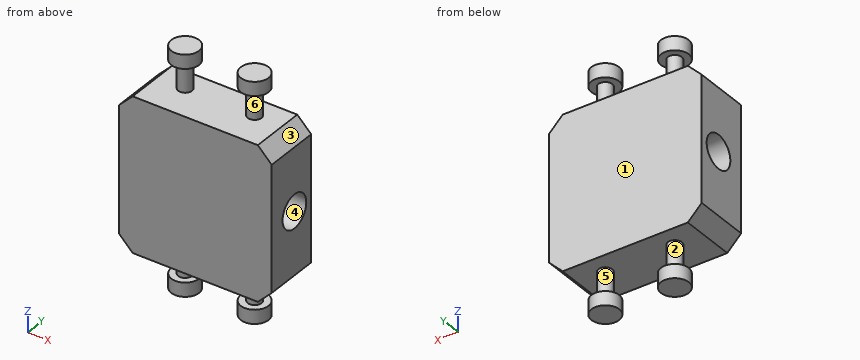
```python
from build123d import *

# Parameters (mm, degrees)
SKETCH2_W           = 110
SKETCH2_H           = 110
BOSS_EXTRUDE1_DEPTH = 30
CHAMFER1_SIZE       = 10
SKETCH3_R           = 5
BOSS_EXTRUDE2_DEPTH = 20
BOSS_EXTRUDE3_START = 20
SKETCH4_R           = 5
BOSS_EXTRUDE3_DEPTH = 20
SKETCH5_R           = 10
BOSS_EXTRUDE4_DEPTH = 10
BOSS_EXTRUDE5_START = 10
SKETCH6_R           = 10
BOSS_EXTRUDE5_DEPTH = 10
BOSS_EXTRUDE6_DEPTH = 5
BOSS_EXTRUDE7_DEPTH = 5
SKETCH15_R          = 12
CUT_EXTRUDE1_DEPTH  = 200


with BuildPart() as part:
    # Sketch2 → Boss-Extrude1 (new body)
    with BuildSketch(Plane(origin=(0, 0, 0), x_dir=(1, 0, 0), z_dir=(0, 1, 0))):
        with Locations((55, 55)):
            Rectangle(SKETCH2_W, SKETCH2_H)
    extrude(amount=BOSS_EXTRUDE1_DEPTH)

    # Chamfer1
    chamfer1_edges = [part.edges().sort_by_distance(p)[0] for p in [
        (0, 15, -110),
        (110, 15, -110),
        (110, 15, 0),
        (0, 15, 0),
    ]]
    chamfer(chamfer1_edges, length=CHAMFER1_SIZE)

    # Sketch3 → Boss-Extrude2 (add)
    with BuildSketch(Plane.XY):
        with Locations(Location((30, 20, 0), (0, 0, 180))):
            Circle(SKETCH3_R)
        with Locations(Location((80, 20, 0), (0, 0, 180))):
            Circle(SKETCH3_R)
    extrude(amount=BOSS_EXTRUDE2_DEPTH)

    # Sketch4 → Boss-Extrude3 (add)
    with BuildSketch(Plane(origin=(0, 0, -110), x_dir=(-1, 0, 0), z_dir=(0, 0, -1)).offset(BOSS_EXTRUDE3_START)):
        with Locations((-80, 20)):
            Circle(SKETCH4_R)
        with Locations((-30, 20)):
            Circle(SKETCH4_R)
    extrude(amount=-BOSS_EXTRUDE3_DEPTH)

    # Sketch5 → Boss-Extrude4 (add)
    with BuildSketch(Plane(origin=(0, 0, -130), x_dir=(-1, 0, 0), z_dir=(0, 0, -1))):
        with Locations((-80, 20)):
            Circle(SKETCH5_R)
        with Locations((-30, 20)):
            Circle(SKETCH5_R)
    extrude(amount=BOSS_EXTRUDE4_DEPTH)

    # Sketch6 → Boss-Extrude5 (add)
    with BuildSketch(Plane.XY.offset(20).offset(BOSS_EXTRUDE5_START)):
        with Locations(Location((30, 20, 0), (0, 0, 180))):
            Circle(SKETCH6_R)
        with Locations(Location((80, 20, 0), (0, 0, 180))):
            Circle(SKETCH6_R)
    extrude(amount=-BOSS_EXTRUDE5_DEPTH)

    # Sketch9 → Boss-Extrude6 (add)
    with BuildSketch(Plane(origin=(0, 30, 0), x_dir=(1, 0, 0), z_dir=(0, 1, 0))):
        Polygon((10, 110), (100, 110), (110, 100), (110, 10), (100, 0), (10, 0), (0, 10), (0, 100), align=None)
    extrude(amount=BOSS_EXTRUDE6_DEPTH)

    # Sketch10 → Boss-Extrude7 (add)
    with BuildSketch(Plane.XZ):
        Polygon((10, 0), (100, 0), (110, -10), (110, -100), (100, -110), (10, -110), (0, -100), (0, -10), align=None)
    extrude(amount=BOSS_EXTRUDE7_DEPTH)

    # Sketch15 → Cut-Extrude1 (cut)
    with BuildSketch(Plane(origin=(110, 0, 0), x_dir=(0, 0, -1), z_dir=(1, 0, 0))):
        with Locations((55, 18)):
            Circle(SKETCH15_R)
    extrude(amount=-CUT_EXTRUDE1_DEPTH, mode=Mode.SUBTRACT)


solid = part.part
```
Geometry: final body of the model. Coordinates: model frame, mm. Face numbers are marked on the shaded views. A direction names the side the tool comes from. Coordinates: 2 decimals unless noted, no trailing zeros. Order: outer loops, then holes, each group sorted by start corner. A loop starts at its lowest first (then second) coordinate and runs counter-clockwise, first axis right, second up. Notation, with made-up numbers: (27.5, -30.75) -> (31.5, -30.75) arc R20 ccw to (31.5, -14.75) -> close; hole circle Ø9 at (71, -22). An arc over 180 degrees is marked (long way). Answer in a Markdown table with one row per item.
Item 1: Section D-D on z = -102.5. Output: boundary loops of the cut face in (x, y).
Return value:
| item | result |
|---|---|
| outline | (2.5, -5) -> (107.5, -5) -> (107.5, 35) -> (2.5, 35) -> close |
Item 2: Draft query along X for the marked faces 3, 4, 5 and 6. Return one class per face: released by +X, released by -X, zero draft, split by the parting line, or undercut.
Return value:
| item | result |
|---|---|
| face 3 | released by +X |
| face 4 | zero draft |
| face 5 | undercut |
| face 6 | undercut |
Item 3: Section B-B on x = 80. Output: boundary loops of the cut face in (y, z), plus the area to 3 significant figures.
Return value:
| item | result |
|---|---|
| outline | (-5, -110) -> (15, -110) -> (15, -130) -> (10, -130) -> (10, -140) -> (30, -140) -> (30, -130) -> (25, -130) -> (25, -110) -> (35, -110) -> (35, 0) -> (25, 0) -> (25, 20) -> (30, 20) -> (30, 30) -> (10, 30) -> (10, 20) -> (15, 20) -> (15, 0) -> (-5, 0) -> close; hole circle Ø24 at (18, -55) |
| area | 4,750 mm² |
Item 4: Section C-C on y = -1.5. Output: boundary loops of the cut face in (x, z).
Return value:
| item | result |
|---|---|
| outline | (0, -100) -> (10, -110) -> (100, -110) -> (110, -100) -> (110, -10) -> (100, 0) -> (10, 0) -> (0, -10) -> close |
Item 5: Section A-A on z = -55. Output: boundary loops of the cut face in (x, y).
Return value:
| item | result |
|---|---|
| outline | (0, -5) -> (110, -5) -> (110, 6) -> (0, 6) -> close; (0, 30) -> (110, 30) -> (110, 35) -> (0, 35) -> close |
Item 6: Contact query for flat-ended pins moving along their axis: P1, Ø20, axis at x = 57, y = 13.5, coming from the -Z side; P2, Ø3, axis at x = 31, z = -120.5, coming from the +Y side; P3, Ø4, axis at x = 15.5, y = 19.5, coming from the +Z side. Output: stop coordinate, or through.
Return value:
| item | result |
|---|---|
| P1 | stops at z = -110 |
| P2 | stops at y = 25 |
| P3 | stops at z = 0 |
Item 7: Ray query, L1, parallel to Y at x = 82, z = -55; L2, parallel to Z at x = 26, y = 16; L3, parallel to X at y = 19.5, z = 19. Return the intervals inside material, ascending.
Return value:
| item | result |
|---|---|
| L1 | y = -5 to 6, 30 to 35 |
| L2 | z = -140 to -130, -110 to -66.83, -43.17 to 0, 20 to 30 |
| L3 | x = 25.03 to 34.97, 75.03 to 84.97 |
Item 8: Access query for the marked faces 1 and 2. Directions: +Z, -Z, +X, -X, +Y, -Y. A direction counts if a zero-diameter tool reaches every point of the face in a straight line with its end or side. Return the directions, or none.
Return value:
| item | result |
|---|---|
| face 1 | +Z, -Z, +X, -X, +Y |
| face 2 | none |
